from build123d import *

# Parameters (mm, degrees)
SKETCH_1_R          = 15
EXTRUDE_1_DEPTH     = 3
SKETCH_2_R          = 6
EXTRUDE_2_DEPTH     = 16.5
FILLET_1_R          = 3
FILLET_2_R          = 1
FILLET_3_R          = 1
SKETCH_3_R          = 6
SKETCH_3_R_2        = 5.5
CUT_EXTRUDE_1_DEPTH = 4
CHAMFER_1_SIZE      = 1


with BuildPart() as part:
    # 草图1 → 凸台-拉伸1 (new body)
    with BuildSketch(Plane.XY):
        Circle(SKETCH_1_R)
    extrude(amount=EXTRUDE_1_DEPTH)

    # 草图2 → 凸台-拉伸2 (add)
    with BuildSketch(Plane.XY.offset(3)):
        Circle(SKETCH_2_R)
    extrude(amount=EXTRUDE_2_DEPTH)

    # 圆角1
    fillet_1_edges = [part.edges().sort_by_distance(p)[0] for p in [
        (-6, 0, 3),
    ]]
    fillet(fillet_1_edges, radius=FILLET_1_R)

    # 圆角2
    fillet_2_edges = [part.edges().sort_by_distance(p)[0] for p in [
        (-15, 0, 3),
    ]]
    fillet(fillet_2_edges, radius=FILLET_2_R)

    # 圆角3
    fillet_3_edges = [part.edges().sort_by_distance(p)[0] for p in [
        (-6, 0, 19.5),
    ]]
    fillet(fillet_3_edges, radius=FILLET_3_R)

    # 草图3 → 切除-拉伸1 (cut)
    with BuildSketch(Plane(origin=(0, 0, 13), x_dir=(-1, 0, 0), z_dir=(0, 0, -1))):
        Circle(SKETCH_3_R)
        Circle(SKETCH_3_R_2, mode=Mode.SUBTRACT)
    extrude(amount=-CUT_EXTRUDE_1_DEPTH, mode=Mode.SUBTRACT)

    # 倒角1
    # the kernel refuses this chamfer: 1 mm, written as the material it adds along each edge
    with BuildSketch(Plane(origin=(0, 0, 13), x_dir=(-1, 0, 0), z_dir=(0, -1, 0))) as chamfer_1_piece_1_section:
        Polygon((5.5 + CHAMFER_1_SIZE, 0), (5.5, -CHAMFER_1_SIZE), (5.5, 0), align=None)
    chamfer_1_piece_1 = revolve(axis=Axis((0, 0, 13), (0, 0, -1)), mode=Mode.PRIVATE)
    chamfer_1_piece_1 = chamfer_1_piece_1 & Plane(origin=(0, 0, 13.746832488), x_dir=(1, 0, 0), z_dir=(0, 0, -1)) * Cylinder(6, 26, mode=Mode.PRIVATE)
    add(chamfer_1_piece_1)
    with BuildSketch(Plane(origin=(0, 0, 17), x_dir=(-1, 0, 0), z_dir=(0, -1, 0))) as chamfer_1_piece_2_section:
        Polygon((5.5, CHAMFER_1_SIZE), (5.5 + CHAMFER_1_SIZE, 0), (5.5, 0), align=None)
    chamfer_1_piece_2 = revolve(axis=Axis((0, 0, 17), (0, 0, -1)), mode=Mode.PRIVATE)
    chamfer_1_piece_2 = chamfer_1_piece_2 & Plane(origin=(0, 0, 16.253167512), x_dir=(1, 0, 0), z_dir=(0, 0, -1)) * Cylinder(6, 26, mode=Mode.PRIVATE)
    add(chamfer_1_piece_2)


solid = part.part
CAD build for the part. Positions are in the model's coordinates, mm. Round coordinates to 2 decimals unless told otherwise and drop trailing zeros. Write each loop counter-clockwise with the first axis right and the second up, starting at its lowest first coordinate (ties: lowest second). Pieces come first, ordered by that corner, then holes.
(1) Slice it at C-C, the plane z = 9. Write the cut outline in (x, y), and give its area (3 significant figures).
(2) Probe line 1 along Z through (x, y) = (-8, -8.25); line 2 along X through (y, z) = (0, 7.5); line 3 along X through (y, z) = (-5, 10.5). List the from-to ranges inside material, lowest first.
(3) Mould opens along Z. For faces 1 (the face through (-14.985, 0.66, 0.986)), 2 (the face through (1.19, -5.37, 14.99)), 3 (the face through (0, 0, 0)), 4 (the face through (0, 0, 19.5)) say: pulls with the +Z half, pulls with the -Z half, needs draft (parallel to the pull), parting line crosses it, or undercut.
(4) Slice it at D-D, the plane z = 14.5. Write the cut outline in (x, y), and give its area (3 significant figures).
(5) Slice it at A-A, the plane y = 0. Write the cut outline in (x, z), and give its area (3 significant figures).
(6) Drop flat-ended pins along their axis: P1, Ø2, axis at x = 10.5, z = 3, coming from the -Y side; P2, Ø1, axis at x = 3.5, z = 17, coming from the -Y side; P3, Ø8, axis at x = -5, z = 8, coming from the -Y side. Give the stop position or say it passes through.
From the geometry:
1. outline: circle Ø12 at (0, 0)
1. area: 113 mm2
2. line 1: z = 0 to 3
2. line 2: x = -6 to 6
2. line 3: x = -3.32 to 3.32
3. face 1: needs draft
3. face 2: undercut
3. face 3: pulls with the -Z half
3. face 4: pulls with the +Z half
4. outline: circle Ø11 at (0, 0)
4. area: 95.0 mm2
5. outline: (-15, 0) - (15, 0) - (15, 2) arc R1 ccw to (14, 3) - (9, 3) arc R3 cw to (6, 6) - (6, 13.5) - (5.5, 14) - (5.5, 16) - (6, 16.5) - (6, 18.5) arc R1 ccw to (5, 19.5) - (-5, 19.5) arc R1 ccw to (-6, 18.5) - (-6, 16.5) - (-5.5, 16) - (-5.5, 14) - (-6, 13.5) - (-6, 6) arc R3 cw to (-9, 3) - (-14, 3) arc R1 ccw to (-15, 2) - close
5. area: 289 mm2
6. P1: stops at y = -11.33
6. P2: stops at y = -5.2
6. P3: stops at y = -5.92
